Input: part model. Units: mm. Frame: model coordinates. Face numbers are marked on the shaded views. A direction names the side the tool comes from. Coordinates: 2 decimals unless noted, no trailing zeros. Loops run counter-clockwise (first coordinate to the right, second up) from the corner with the lowest first, then second, coordinate; pieces in that order, holes last. Notation, with made-up numbers: (28.25, -13) -> (35.25, -13) arc R32 cw to (35.25, 23) -> close; hole circle Ø9 at (89, 69.5). An arc over 180 degrees is marked (long way). Answer as a JSON object with one key per item and string values.
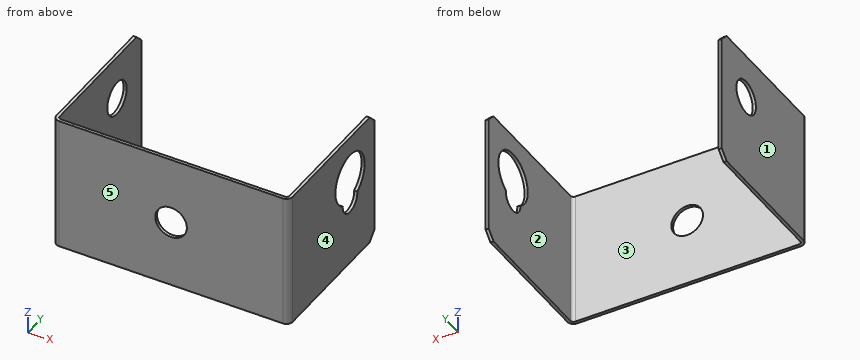
from build123d import *

# Parameters (mm, degrees)
BASE_FLANGE1_DEPTH = 32
CUT_EXTRUDE1_DEPTH = 10
SKETCH7_R          = 4
CUT_EXTRUDE2_DEPTH = 10
SKETCH8_R          = 3.75
CUT_EXTRUDE3_DEPTH = 10
CHAMFER1_SIZE      = 2


# Sheet-metal steps are written as plain solids
with BuildPart() as part:
    # Sketch1 → Base-Flange1 (new body)
    with BuildSketch(Plane.XY):
        with BuildLine():
            Line((56, 35), (56, 1.4732))
            ThreePointArc((56, 1.4732), (55.56850971, 0.43149029), (54.5268, 0))
            Line((54.5268, 0), (1.4732, 0))
            ThreePointArc((1.4732, 0), (0.43149029, 0.43149029), (0, 1.4732))
            Line((0, 1.4732), (0, 35))
            Line((0, 35), (0.7366, 35))
            Line((0.7366, 35), (0.7366, 1.4732))
            ThreePointArc((0.7366, 1.4732), (0.952345145, 0.952345145), (1.4732, 0.7366))
            Line((1.4732, 0.7366), (54.5268, 0.7366))
            ThreePointArc((54.5268, 0.7366), (55.047654855, 0.952345145), (55.2634, 1.4732))
            Line((55.2634, 1.4732), (55.2634, 35))
            Line((55.2634, 35), (56, 35))
        make_face()
    extrude(amount=BASE_FLANGE1_DEPTH)

    # Sketch6 → Cut-Extrude1 (cut)
    with BuildSketch(Plane(origin=(56, 0, 0), x_dir=(0, 0, -1), z_dir=(1, 0, 0))):
        with BuildLine():
            ThreePointArc((-16.295454545, 27.985415651), (-27.5, 25), (-16.295454545, 22.014584349))
            ThreePointArc((-16.295454545, 22.014584349), (-13, 25), (-16.295454545, 27.985415651))
        make_face()
    extrude(amount=-CUT_EXTRUDE1_DEPTH, mode=Mode.SUBTRACT)

    # Sketch7 → Cut-Extrude2 (cut)
    with BuildSketch(Plane.ZY):
        with Locations((21.5, 25)):
            Circle(SKETCH7_R)
    extrude(amount=-CUT_EXTRUDE2_DEPTH, mode=Mode.SUBTRACT)

    # Sketch8 → Cut-Extrude3 (cut)
    with BuildSketch(Plane(origin=(0, 0.7366, 0), x_dir=(1, 0, 0), z_dir=(0, 1, 0))):
        with Locations(Location((28, -16, 0), (0, 0, 270))):
            Circle(SKETCH8_R)
    extrude(amount=-CUT_EXTRUDE3_DEPTH, mode=Mode.SUBTRACT)

    # Chamfer1
    chamfer1_edges = [part.edges().sort_by_distance(p)[0] for p in [
        (0.3683, 35, 0),
        (55.6317, 35, 0),
        (0.3683, 35, 32),
        (55.6317, 35, 32),
    ]]
    chamfer(chamfer1_edges, length=CHAMFER1_SIZE)


solid = part.part
1. Pin query (flat end, axial travel): P1, Ø16, axis at x = 18.5, z = 18.5, coming from the +Y side. Return the tip coordinate at first contact, or that it passes through.
Reply:
{"P1": "stops at y = 0.74"}
2. Mould query, pull axis X, two halves, no side actions, for the marked faces 3, 4 and 5. Classes: pulls with the +X half, pulls with the -X half, needs draft (parallel to the pull), parting line crosses it, or undercut.
Reply:
{"face 3": "undercut", "face 4": "pulls with the +X half", "face 5": "needs draft"}
3. Section query B-B (y = 25). Return loops of the section in (x, z).
Reply:
{"outline": "(0, 0) -> (0.74, 0) -> (0.74, 17.5) -> (0, 17.5) -> close; (0, 25.5) -> (0.74, 25.5) -> (0.74, 32) -> (0, 32) -> close; (55.26, 0) -> (56, 0) -> (56, 13) -> (55.26, 13) -> close; (55.26, 27.5) -> (56, 27.5) -> (56, 32) -> (55.26, 32) -> close"}
4. Section query A-A (x = 28). Return loops of the section in (y, z), plus the area to 3 significant figures.
Reply:
{"outline": "(0, 0) -> (0.74, 0) -> (0.74, 12.25) -> (0, 12.25) -> close; (0, 19.75) -> (0.74, 19.75) -> (0.74, 32) -> (0, 32) -> close", "area": "18.0 mm2"}
5. Section query C-C (z = 3). Return loops of the section in (x, y).
Reply:
{"outline": "(0, 1.47) arc R1.47 ccw to (1.47, 0) -> (54.53, 0) arc R1.47 ccw to (56, 1.47) -> (56, 35) -> (55.26, 35) -> (55.26, 1.47) arc R0.74 cw to (54.53, 0.74) -> (1.47, 0.74) arc R0.74 cw to (0.74, 1.47) -> (0.74, 35) -> (0, 35) -> close"}
6. Access query for the marked faces 1 and 2. Directions: +Z, -Z, +X, -X, +Y, -Y. A direction counts if a zero-diameter tool reaches every point of the face in a straight line with its end or side. Return the directions, or none.
Reply:
{"face 1": "+Z, -Z, -X, +Y, -Y", "face 2": "+Z, -Z, +Y"}
7. Section query D-D (z = 19). Return loops of the section in (x, y), plus the area to 3 significant figures.
Reply:
{"outline": "(0, 1.47) arc R1.47 ccw to (1.47, 0) -> (25.75, 0) -> (25.75, 0.74) -> (1.47, 0.74) arc R0.74 cw to (0.74, 1.47) -> (0.74, 21.88) -> (0, 21.88) -> close; (0, 28.12) -> (0.74, 28.12) -> (0.74, 35) -> (0, 35) -> close; (30.25, 0) -> (54.53, 0) arc R1.47 ccw to (56, 1.47) -> (56, 19.55) -> (55.26, 19.55) -> (55.26, 1.47) arc R0.74 cw to (54.53, 0.74) -> (30.25, 0.74) -> close; (55.26, 30.45) -> (56, 30.45) -> (56, 35) -> (55.26, 35) -> close", "area": "75.1 mm2"}
8. Line query: line 1 along X through (y, z) = (10.5, 26.5); line 2 along Y through (x, z) = (44.5, 4.5); line 3 along Y through (x, z) = (55, 21). Output: solid intervals per line, ascending.
Reply:
{"line 1": "x = 0 to 0.74, 55.26 to 56", "line 2": "y = 0 to 0.74", "line 3": "y = 0.08 to 0.91"}
